from build123d import *

# Parameters (mm, degrees)
SKETCH1_W           = 175
SKETCH1_H           = 51
BOSS_EXTRUDE1_DEPTH = 17
CUT_EXTRUDE3_DEPTH  = 52
SKETCH7_W           = 4.75
SKETCH7_H           = 4.75
CUT_EXTRUDE5_DEPTH  = 145
SKETCH10_W          = 10.05
SKETCH10_H          = 24
CUT_EXTRUDE6_DEPTH  = 16
SKETCH11_W          = 10.05
SKETCH11_H          = 8.05
CUT_EXTRUDE7_DEPTH  = 8


with BuildPart() as part:
    # Sketch1 → Boss-Extrude1 (new body)
    with BuildSketch(Plane(origin=(0, 0, 0), x_dir=(0, 0, -1), z_dir=(1, 0, 0))):
        with Locations((22.937921078, 5.057266603)):
            Rectangle(SKETCH1_W, SKETCH1_H)
    extrude(amount=BOSS_EXTRUDE1_DEPTH)

    # Sketch6 → Cut-Extrude3 (cut, through all)
    with BuildSketch(Plane(origin=(0, 30.557266603, 0), x_dir=(1, 0, 0), z_dir=(0, 1, 0))):
        Polygon((12.5, -60.062078922), (17, -60.062078922), (17, -57.062078922), (14.5, -57.062078922), (7.75, -57.062078922), (7.75, -62.062078922), (12.5, -62.062078922), align=None)
    extrude(amount=-CUT_EXTRUDE3_DEPTH, mode=Mode.SUBTRACT)

    # Sketch7 → Cut-Extrude5 (cut)
    with BuildSketch(Plane(origin=(0, 0, -110.437921078), x_dir=(-1, 0, 0), z_dir=(0, 0, -1))):
        with Locations((-14.625, 0.432266603)):
            Rectangle(SKETCH7_W, SKETCH7_H)
        with Locations((-14.625, 18.432266603)):
            Rectangle(SKETCH7_W, SKETCH7_H)
    extrude(amount=-CUT_EXTRUDE5_DEPTH, mode=Mode.SUBTRACT)

    # Sketch10 → Cut-Extrude6 (cut)
    with BuildSketch(Plane(origin=(0, 0, -110.437921078), x_dir=(-1, 0, 0), z_dir=(0, 0, -1))):
        with Locations((-11.975, 9.557266603)):
            Rectangle(SKETCH10_W, SKETCH10_H)
    extrude(amount=-CUT_EXTRUDE6_DEPTH, mode=Mode.SUBTRACT)

    # Sketch11 → Cut-Extrude7 (cut)
    with BuildSketch(Plane(origin=(0, -2.442733397, 0), x_dir=(1, 0, 0), z_dir=(0, 1, 0))):
        with Locations((11.975, 98.462921078)):
            Rectangle(SKETCH11_W, SKETCH11_H)
    extrude(amount=-CUT_EXTRUDE7_DEPTH, mode=Mode.SUBTRACT)


solid = part.part
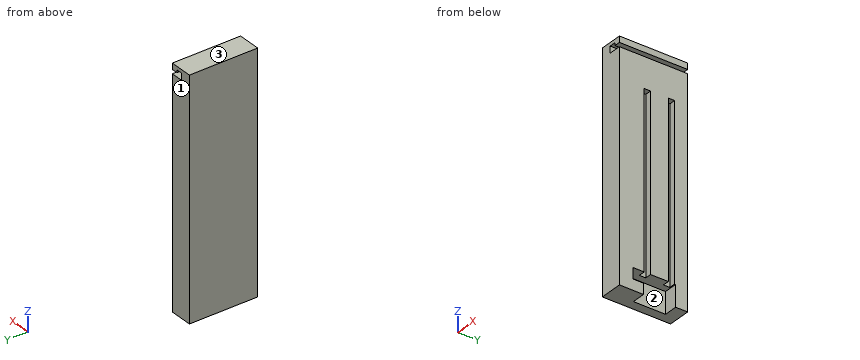
Could you check a few things on this model? Use its own coordinates, in mm. Face numbers are marked on the shaded views. Give positions to 0.01 mm unless a question says otherwise; leave off trailing zeros. Order: outer loops, then holes, each group sorted by start corner. A loop starts at its lowest first (then second) coordinate and runs counter-clockwise, first axis right, second up.
1. Will these pins go through, and if not, where does the flat tip stop? P1, Ø13, axis at y = 6, z = -103.5, coming from the +X side; P2, Ø5, axis at x = 10.5, y = 14.5, coming from the -Z side.
2. Suppose I cut it at B-B (x = 14.75). List the corners of the cut face in (y, z) for me.
3. I need wall thicknesses on L1, parallel to Y at x = 14.25, z = -43; L2, parallel to Z at x = 13.25, y = -8; L3, parallel to Z at x = 10.5, y = -16. Which ranges of each line are inside material? Lowest first, please.
4. We'd pull the mould along Y, two halves only. Please class the marked faces 1, 2 and 3: pulls with the +Y half, pulls with the -Y half, needs draft (parallel to the pull), parting line crosses it, or undercut.
5. Suppose I cut it at C-C (z = 9). List the corners of the cut face in (x, y) for me.
6. Suppose I cut it at D-D (y = -8.5). List the corners of the cut face in (x, z) for me, plus the area to 3 significant figures.
7. Suppose I cut it at A-A (y = 18). List the corners of the cut face in (x, z) for me.
Solved:
1. P1: stops at x = 6.95
1. P2: stops at z = -94.44
2. outline: (-20.44, -110.44) - (-2.44, -110.44) - (-2.44, -102.49) - (-10.44, -102.49) - (-10.44, -94.44) - (-1.94, -94.44) - (-1.94, 34.56) - (2.81, 34.56) - (2.81, -94.44) - (16.06, -94.44) - (16.06, 34.56) - (20.81, 34.56) - (20.81, -94.44) - (21.56, -94.44) - (21.56, -110.44) - (30.56, -110.44) - (30.56, 57.06) - (-20.44, 57.06) - close; (-20.44, 60.06) - (30.56, 60.06) - (30.56, 64.56) - (-20.44, 64.56) - close
3. L1: y = -20.44 to -1.94, 2.81 to 16.06, 20.81 to 30.56
3. L2: z = -110.44 to -102.49, -94.44 to 57.06, 60.06 to 64.56
3. L3: z = -110.44 to 57.06, 62.06 to 64.56
4. face 1: pulls with the +Y half
4. face 2: undercut
4. face 3: needs draft
5. outline: (0, -20.44) - (17, -20.44) - (17, -1.94) - (12.25, -1.94) - (12.25, 2.81) - (17, 2.81) - (17, 16.06) - (12.25, 16.06) - (12.25, 20.81) - (17, 20.81) - (17, 30.56) - (0, 30.56) - close
6. outline: (0, -110.44) - (17, -110.44) - (17, -102.49) - (6.95, -102.49) - (6.95, -94.44) - (17, -94.44) - (17, 57.06) - (7.75, 57.06) - (7.75, 62.06) - (12.5, 62.06) - (12.5, 60.06) - (17, 60.06) - (17, 64.56) - (0, 64.56) - close
6. area: 2,860 mm2
7. outline: (0, -110.44) - (6.95, -110.44) - (6.95, -94.44) - (12.25, -94.44) - (12.25, 34.56) - (17, 34.56) - (17, 57.06) - (7.75, 57.06) - (7.75, 62.06) - (12.5, 62.06) - (12.5, 60.06) - (17, 60.06) - (17, 64.56) - (0, 64.56) - close
